For this review, take the finished solid that the model builds, in its own axes (mm). Face numbers are marked on the shaded views. A direction names the side the tool comes from. Give positions to 0.01 mm unless a question says otherwise; leave off trailing zeros. Write each loop counter-clockwise with the first axis right and the second up, starting at its lowest first coordinate (ties: lowest second). Pieces come first, ordered by that corner, then holes. Notation, with made-up numbers: M 84.25,16 L 104.25,16 A15 cw 104.25,43 Z; hole C 2,32.5 d3. An arc over 180 degrees is marked long. Use one line per item in the form item = value. Start each with the question number.
Q1. Clearance check with flat-ended pins moving along their axes: pin 1 Ø2.5 at (x, z) = (12.5, 1) entering from +Y; pin 2 Ø0.7 at (x, z) = (6, 30) entering from -Y; pin 3 Ø1.5 at (x, z) = (11, -13) entering from -Y; pin 4 Ø1.8 at (x, y) = (4.5, -9.83) entering from +Z. State where each tip first meets the part, or that it passes through.
Q2. Consider section D-D on y = -7. Write out the cut boundary in (x, z).
Q3. Consider section C-C on z = 1. Write out the cut boundary in (x, y).
Q4. For probe 1 along Y at (x, z) = (12.5, 29.9); probe 2 along Z at (x, y) = (11.5, 2); probe 3 along Z at (x, y) = (12.5, 45.2), list the stretches that pass through material, from the lowest coordinate up. Write a range as [from, to].
Q5. Consider section B-B on y = 15. Write out the cut boundary in (x, z), and give its area (3 significant figures).
Q6. Consider section A-A on x = 12.5. Write out the cut boundary in (y, z), and give its area (3 significant figures).
Q7. Mouldability with a two-part tool opening along Z and no side actions: class the marked faces 3, 4, 5 and 6 as released by +Z, released by -Z, zero draft, split by the parting line, or undercut.
Q8. Tool access review of the marked faces 1 and 2: name each direction out of +Z, -Z, +X, -X, +Y, -Y from which nothing blocks a thin tool from reaching the whole face with its end or side.
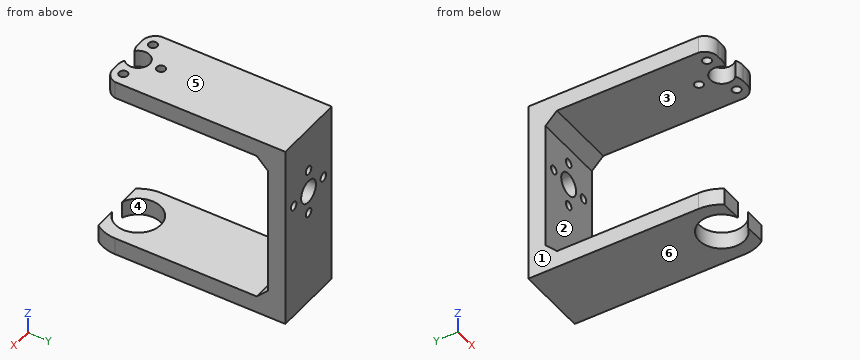
```python
from build123d import *

# Parameters (mm, degrees)
SALIENTE_EXTRUIR1_DEPTH = 25
CORTAR_EXTRUIR2_REACH   = 67.2
CORTAR_EXTRUIR3_REACH   = 72
CROQUIS4_R              = 1.5
CROQUIS4_R_2            = 4
CHAFL_N1_SIZE           = 4
CORTAR_EXTRUIR5_REACH   = 67.2
CROQUIS8_R              = 1.5


with BuildPart() as part:
    # Croquis1 → Saliente-Extruir1 (new body)
    with BuildSketch(Plane(origin=(0, 0, 0), x_dir=(0, 0, -1), z_dir=(1, 0, 0))):
        Polygon((-26.6, -20.333615037), (-26.6, 43.666384963), (26.6, 43.666384963), (26.6, -20.333615037), (32.6, -20.333615037), (32.6, 49.666384963), (-32.6, 49.666384963), (-32.6, -20.333615037), align=None)
    extrude(amount=SALIENTE_EXTRUIR1_DEPTH)

    # Croquis3 → Cortar-Extruir2 (cut, up to next)
    with BuildSketch(Plane(origin=(0, 0, -32.6), x_dir=(-1, 0, 0), z_dir=(0, 0, -1)), mode=Mode.PRIVATE) as cortar_extruir2_sk1:
        with BuildLine():
            Line((-15.246347098, -17.240880228), (-22.56888387, -17.240880228))
            ThreePointArc((-22.56888387, -17.240880228), (-24.376679847, -13.731624248), (-25, -9.833615037))
            Line((-25, -9.833615037), (-25, -20.333615037))
            Line((-25, -20.333615037), (0, -20.333615037))
            Line((0, -20.333615037), (0, -9.833615037))
            ThreePointArc((0, -9.833615037), (-0.623320153, -13.731624248), (-2.43111613, -17.240880228))
            Line((-2.43111613, -17.240880228), (-9.753652902, -17.240880228))
            ThreePointArc((-9.753652902, -17.240880228), (-12.5, -1.933615037), (-15.246347098, -17.240880228))
        make_face()
    cortar_extruir2_tool1 = extrude(cortar_extruir2_sk1.sketch, amount=-CORTAR_EXTRUIR2_REACH, mode=Mode.PRIVATE) & part.part
    add(cortar_extruir2_tool1.solids().sort_by_distance((12.5, -12.457644, -32.6))[0], mode=Mode.SUBTRACT)

    # Croquis4 → Cortar-Extruir3 (cut, up to next)
    with BuildSketch(Plane(origin=(0, 49.666384963, 0), x_dir=(1, 0, 0), z_dir=(0, 1, 0)), mode=Mode.PRIVATE) as cortar_extruir3_sk1:
        with Locations((12.5, -1)):
            Circle(CROQUIS4_R)
    cortar_extruir3_tool1 = extrude(cortar_extruir3_sk1.sketch, amount=-CORTAR_EXTRUIR3_REACH, mode=Mode.PRIVATE) & part.part
    add(cortar_extruir3_tool1.solids().sort_by_distance((12.5, 49.666385, 1))[0], mode=Mode.SUBTRACT)
    # Croquis4 → Cortar-Extruir3 (cut, up to next)
    with BuildSketch(Plane(origin=(0, 49.666384963, 0), x_dir=(1, 0, 0), z_dir=(0, 1, 0)), mode=Mode.PRIVATE) as cortar_extruir3_sk2:
        with Locations((4.5, -9)):
            Circle(CROQUIS4_R)
    cortar_extruir3_tool2 = extrude(cortar_extruir3_sk2.sketch, amount=-CORTAR_EXTRUIR3_REACH, mode=Mode.PRIVATE) & part.part
    add(cortar_extruir3_tool2.solids().sort_by_distance((4.5, 49.666385, 9))[0], mode=Mode.SUBTRACT)
    # Croquis4 → Cortar-Extruir3 (cut, up to next)
    with BuildSketch(Plane(origin=(0, 49.666384963, 0), x_dir=(1, 0, 0), z_dir=(0, 1, 0)), mode=Mode.PRIVATE) as cortar_extruir3_sk3:
        with Locations((12.5, -17)):
            Circle(CROQUIS4_R)
    cortar_extruir3_tool3 = extrude(cortar_extruir3_sk3.sketch, amount=-CORTAR_EXTRUIR3_REACH, mode=Mode.PRIVATE) & part.part
    add(cortar_extruir3_tool3.solids().sort_by_distance((12.5, 49.666385, 17))[0], mode=Mode.SUBTRACT)
    # Croquis4 → Cortar-Extruir3 (cut, up to next)
    with BuildSketch(Plane(origin=(0, 49.666384963, 0), x_dir=(1, 0, 0), z_dir=(0, 1, 0)), mode=Mode.PRIVATE) as cortar_extruir3_sk4:
        with Locations((20.5, -9)):
            Circle(CROQUIS4_R)
    cortar_extruir3_tool4 = extrude(cortar_extruir3_sk4.sketch, amount=-CORTAR_EXTRUIR3_REACH, mode=Mode.PRIVATE) & part.part
    add(cortar_extruir3_tool4.solids().sort_by_distance((20.5, 49.666385, 9))[0], mode=Mode.SUBTRACT)
    # Croquis4 → Cortar-Extruir3 (cut, up to next)
    with BuildSketch(Plane(origin=(0, 49.666384963, 0), x_dir=(1, 0, 0), z_dir=(0, 1, 0)), mode=Mode.PRIVATE) as cortar_extruir3_sk5:
        with Locations((12.5, -9)):
            Circle(CROQUIS4_R_2)
    cortar_extruir3_tool5 = extrude(cortar_extruir3_sk5.sketch, amount=-CORTAR_EXTRUIR3_REACH, mode=Mode.PRIVATE) & part.part
    add(cortar_extruir3_tool5.solids().sort_by_distance((12.5, 49.666385, 9))[0], mode=Mode.SUBTRACT)

    # Chaflán1
    chafl_n1_edges = [part.edges().sort_by_distance(p)[0] for p in [
        (12.5, 43.666384963, -26.6),
        (12.5, 43.666384963, 26.6),
    ]]
    chamfer(chafl_n1_edges, length=CHAFL_N1_SIZE)

    # Croquis8 → Cortar-Extruir5 (cut, up to next)
    with BuildSketch(Plane.XY.offset(32.6), mode=Mode.PRIVATE) as cortar_extruir5_sk1:
        with Locations((4.5, -9.833615037)):
            Circle(CROQUIS8_R)
    cortar_extruir5_tool1 = extrude(cortar_extruir5_sk1.sketch, amount=-CORTAR_EXTRUIR5_REACH, mode=Mode.PRIVATE) & part.part
    add(cortar_extruir5_tool1.solids().sort_by_distance((4.5, -9.833615, 32.6))[0], mode=Mode.SUBTRACT)
    # Croquis8 → Cortar-Extruir5 (cut, up to next)
    with BuildSketch(Plane.XY.offset(32.6), mode=Mode.PRIVATE) as cortar_extruir5_sk2:
        with Locations((12.5, -1.833615037)):
            Circle(CROQUIS8_R)
    cortar_extruir5_tool2 = extrude(cortar_extruir5_sk2.sketch, amount=-CORTAR_EXTRUIR5_REACH, mode=Mode.PRIVATE) & part.part
    add(cortar_extruir5_tool2.solids().sort_by_distance((12.5, -1.833615, 32.6))[0], mode=Mode.SUBTRACT)
    # Croquis8 → Cortar-Extruir5 (cut, up to next)
    with BuildSketch(Plane.XY.offset(32.6), mode=Mode.PRIVATE) as cortar_extruir5_sk3:
        with Locations((20.5, -9.833615037)):
            Circle(CROQUIS8_R)
    cortar_extruir5_tool3 = extrude(cortar_extruir5_sk3.sketch, amount=-CORTAR_EXTRUIR5_REACH, mode=Mode.PRIVATE) & part.part
    add(cortar_extruir5_tool3.solids().sort_by_distance((20.5, -9.833615, 32.6))[0], mode=Mode.SUBTRACT)
    # Croquis8 → Cortar-Extruir5 (cut, up to next)
    with BuildSketch(Plane.XY.offset(32.6), mode=Mode.PRIVATE) as cortar_extruir5_sk4:
        with BuildLine():
            Line((4.605097731, -13.578746505), (6.89606083, -13.578746505))
            ThreePointArc((6.89606083, -13.578746505), (8.414491828, -13.385028449), (9.836162211, -12.817566818))
            ThreePointArc((9.836162211, -12.817566818), (12.5, -5.833615037), (15.163837789, -12.817566818))
            ThreePointArc((15.163837789, -12.817566818), (16.585508172, -13.385028449), (18.10393917, -13.578746505))
            Line((18.10393917, -13.578746505), (20.394902269, -13.578746505))
            ThreePointArc((20.394902269, -13.578746505), (23.36276913, -12.524270715), (25, -9.833615037))
            Line((25, -9.833615037), (25, -20.333615037))
            Line((25, -20.333615037), (0, -20.333615037))
            Line((0, -20.333615037), (0, -9.833615037))
            ThreePointArc((0, -9.833615037), (1.63723087, -12.524270715), (4.605097731, -13.578746505))
        make_face()
    cortar_extruir5_tool4 = extrude(cortar_extruir5_sk4.sketch, amount=-CORTAR_EXTRUIR5_REACH, mode=Mode.PRIVATE) & part.part
    add(cortar_extruir5_tool4.solids().sort_by_distance((12.5, -15.203922, 32.6))[0], mode=Mode.SUBTRACT)


solid = part.part
```
Working result:
q1.pin_1 = through
q1.pin_2 = -13.58
q1.pin_3 = 43.67
q1.pin_4 = -26.6
q2.outline = M 0,-32.6 L 5.13,-32.6 L 5.13,-26.6 L 0,-26.6 Z; M 0,26.6 L 9.68,26.6 L 9.68,32.6 L 0,32.6 Z; M 15.32,26.6 L 25,26.6 L 25,32.6 L 15.32,32.6 Z; M 19.87,-32.6 L 25,-32.6 L 25,-26.6 L 19.87,-26.6 Z
q3.outline = M 0,43.67 L 11,43.67 L 11,49.67 L 0,49.67 Z; M 14,43.67 L 25,43.67 L 25,49.67 L 14,49.67 Z
q4.probe_1 = [-5.83, -3.33], [-0.33, 49.67]
q4.probe_2 = [-32.6, -26.6], [26.6, 32.6]
q4.probe_3 = [-32.6, -0.5], [2.5, 5], [13, 15.5], [18.5, 32.6]
q5.outline = M 0,-32.6 L 25,-32.6 L 25,-26.6 L 0,-26.6 Z; M 0,26.6 L 25,26.6 L 25,32.6 L 0,32.6 Z
q5.area = 300 mm²
q6.outline = M -5.83,26.6 L -3.33,26.6 L -3.33,32.6 L -5.83,32.6 Z; M -1.93,-32.6 L 49.67,-32.6 L 49.67,-0.5 L 43.67,-0.5 L 43.67,-22.6 L 39.67,-26.6 L -1.93,-26.6 Z; M -0.33,26.6 L 39.67,26.6 L 43.67,22.6 L 43.67,18.5 L 49.67,18.5 L 49.67,32.6 L -0.33,32.6 Z; M 43.67,2.5 L 49.67,2.5 L 49.67,5 L 43.67,5 Z; M 43.67,13 L 49.67,13 L 49.67,15.5 L 43.67,15.5 Z
q6.area = 876 mm²
q7.face_3 = undercut
q7.face_4 = zero draft
q7.face_5 = released by +Z
q7.face_6 = released by -Z
q8.face_1 = +Z, -Z, -X, +Y, -Y
q8.face_2 = +X, -X, -Y
